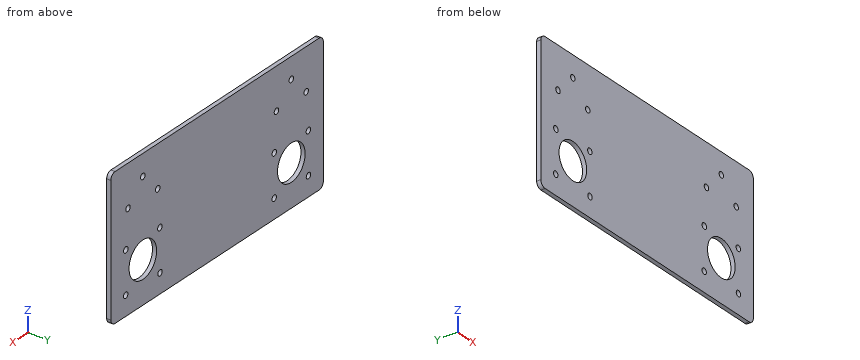
Autodesk Inventor part; units mm, degrees
ref_plane "YZ Plane" through (0, 0, 0) normal (1, 0, 0) x (0, 1, 0)
ref_plane "XZ Plane" through (0, 0, 0) normal (0, 1, 0) x (-1, 0, 0)
ref_plane "XY Plane" through (0, 0, 0) normal (0, 0, 1) x (1, 0, 0)
sketch "Sketch1" plane through (0, 0, 0) normal (0, 1, 0) x (-1, 0, 0)
  circle A0 centre (15.07, -33) radius 6.5
  circle A1 centre (84.93, -33) radius 6.5
  circle A2 centre (15.07, -5.58) radius 1.05
  circle A3 centre (22.07, -12.88) radius 1.05
  circle A4 centre (8.07, -12.88) radius 1.05
  circle A5 centre (23.07, -26.1) radius 1.05
  circle A6 centre (7.07, -26.1) radius 1.05
  circle A7 centre (7, -41) radius 1.05
  circle A8 centre (23.14, -41) radius 1.05
  circle A9 centre (93, -41) radius 1.05
  circle A10 centre (76.86, -41) radius 1.05
  circle A11 centre (76.93, -26.1) radius 1.05
  circle A12 centre (92.93, -26.1) radius 1.05
  circle A13 centre (91.93, -12.88) radius 1.05
  circle A14 centre (77.93, -12.88) radius 1.05
  circle A15 centre (84.93, -5.58) radius 1.05
  arc A16 (100, 0) -> (98, 2) centre (98, 0) ccw
  line L0 (100, 0) -> (100, -46)
  line L1 (2, 2) -> (98, 2)
  arc A17 (2, 2) -> (0, 0) centre (2, 0) ccw
  line L2 (0, -46) -> (0, 0)
  arc A18 (0, -46) -> (2, -48) centre (2, -46) ccw
  line L3 (98, -48) -> (2, -48)
  arc A19 (98, -48) -> (100, -46) centre (98, -46) ccw
  point P0 (0, 0)
extrude "Extrusion1" add sketch "Sketch1" against normal blind 1.5
properties part number "body_bottom_frame"
Design review of the part built by this model. Coordinates are the model's own, in mm. Coordinates: 2 decimals unless noted, no trailing zeros. Order: outer loops, then holes, each group sorted by start corner. A loop starts at its lowest first (then second) coordinate and runs counter-clockwise, first axis right, second up. Notation, with made-up numbers: (62, 79.25) -> (95, 79.25) arc R19 cw to (95, 97.25) -> close; hole circle Ø8 at (55, 26). An arc over 180 degrees is marked (long way). One line per item, written item: value. Start each with the question number.
Q1. For probe 1 along Z at (x, y) = (-84.93, -0.75); probe 2 along X at (y, z) = (-1, -6.5); probe 3 along X at (y, z) = (-0.5, -28), list the stretches that pass through material, from the lowest coordinate up.
Q2. Take a section at C-C, the plane z = -30.5. State the section outline as (x, y) points, then the cut area to 3 significant figures.
Q3. Take a section at A-A, the plane z = -12.88. State the section outline as (x, y) points, then the cut area to 3 significant figures.
Q4. Insertion check: pin 1 Ø1.9 at (x, z) = (-92.93, -26.1) entering from +Y; pin 2 Ø2.5 at (x, z) = (-76.86, -41) entering from +Y. Each pin has a flat end and moves straight along its axis. Give the tip position at first contact, or say it passes through.
Q5. Take a section at B-B, the plane y = -0.5. Give the number of separate pieces and of enclosed holes in the cut face, then the cut area to 3 significant figures.
Values follow:
1. probe 1: z = -48 to -39.5, -26.5 to -6.63, -4.53 to 2
1. probe 2: x = -100 to -85.44, -84.42 to -15.58, -14.56 to 0
1. probe 3: x = -100 to -89.08, -80.78 to -19.22, -10.92 to 0
2. outline: (-100, -1.5) -> (-90.93, -1.5) -> (-90.93, 0) -> (-100, 0) -> close; (-78.93, -1.5) -> (-21.07, -1.5) -> (-21.07, 0) -> (-78.93, 0) -> close; (-9.07, -1.5) -> (0, -1.5) -> (0, 0) -> (-9.07, 0) -> close
2. area: 114 mm2
3. outline: (-100, -1.5) -> (-92.98, -1.5) -> (-92.98, 0) -> (-100, 0) -> close; (-90.88, -1.5) -> (-78.98, -1.5) -> (-78.98, 0) -> (-90.88, 0) -> close; (-76.88, -1.5) -> (-23.12, -1.5) -> (-23.12, 0) -> (-76.88, 0) -> close; (-21.02, -1.5) -> (-9.12, -1.5) -> (-9.12, 0) -> (-21.02, 0) -> close; (-7.02, -1.5) -> (0, -1.5) -> (0, 0) -> (-7.02, 0) -> close
3. area: 137 mm2
4. pin 1: passes through
4. pin 2: stops at y = 0
5. separate pieces: 1
5. enclosed holes: 16
5. area: 4,680 mm2
